Here's how the part is built. I have some questions about the finished solid (model axes, mm). A direction names the side the tool comes from. Round coordinates to 2 decimals unless told otherwise and drop trailing zeros. Write each loop counter-clockwise with the first axis right and the second up, starting at its lowest first coordinate (ties: lowest second). Pieces come first, ordered by that corner, then holes. Notation, with made-up numbers: M 79,-36.75 L 119,-36.75 A36 ccw 119,-2.75 Z; hole C -39,46.25 d9. An arc over 180 degrees is marked long. Use a Markdown table: item, result. Add a question column.
```python
from build123d import *

# Parameters (mm, degrees)
F1_DEPTH = 85.57783
F2_W     = 470.658332
F2_H     = 132.007137
F3_DEPTH = 332.33001
F4_R     = 3.175
F5_DEPTH = 369.06305


with BuildPart() as f1:
    # F0 (on Front) → F1 (new body)
    with BuildSketch(Plane.XZ):
        with BuildLine():
            ThreePointArc((-209.55, 0), (0, 209.55), (209.55, 0))
            Line((209.55, 0), (214.597345, 0))
            ThreePointArc((214.597345, 0), (0, 214.597345), (-214.597345, 0))
            Line((-214.597345, 0), (-209.55, 0))
        make_face()
    extrude(amount=F1_DEPTH)

    # F2 (on Top) → F3 (cut)
    with BuildSketch(Plane.XY):
        with Locations((5.359113, -37.707031)):
            Rectangle(F2_W, F2_H)
        Polygon((-61.859035, -72.326824), (-61.859035, -21.526824), (-31.379035, -21.526824), (-17.515417, -38.048841), (0, -38.048841), (13.863618, -21.526824), (44.343618, -21.526824), (44.343618, -72.326824), (13.863618, -72.326824), (0, -55.804808), (-17.515417, -55.804808), (-31.379035, -72.326824), align=None, mode=Mode.SUBTRACT)
    extrude(amount=F3_DEPTH, mode=Mode.SUBTRACT)

    # F4 (on Top) → F5 (cut)
    with BuildSketch(Plane.XY):
        with Locations((-51.647099, -30.972526)):
            Circle(F4_R)
        with Locations((-51.647099, -64.446411)):
            Circle(F4_R)
        with Locations((-33.92563, -47.118752)):
            Circle(F4_R)
        with Locations((9.262242, -47.118752)):
            Circle(F4_R)
        with Locations((33.022132, -30.972526)):
            Circle(F4_R)
        with Locations((32.234513, -64.446411)):
            Circle(F4_R)
    extrude(amount=F5_DEPTH, mode=Mode.SUBTRACT)


solid = f1.part
```
Item 1: Imagine slicing it at D-D on x = -23.5. List the corners of the cut face in (y, z) for me.
Item 2: Imagine slicing it at B-B on y = -62.5. List the corners of the cut face in (x, z) for me, plus the area to 3 significant figures.
Item 3: For pin 1 Ø7.5 at (x, y) = (-33.93, -47.12) entering from +Z; pin 2 Ø1.5 at (x, z) = (-24, 206) entering from -Y; pin 3 Ø6.5 at (x, z) = (-9, 212.5) entering from +Y; pin 4 Ø1.7 at (x, z) = (-8, 211.5) entering from -Y, each with a flat end and sliding along its axis, tell me the tip position at first contact or that it passes through.
Item 4: If we mould it in two halves opening along Y, with no side actions, what happens to faces 4 (the face through (35.17, -65.66, 209.54)), 5 (the face through (29, -21.527, 209)), 6 (the face through (7.03, -64.18, 211.81))? For each: +Y half, -Y half, draft (parallel to the pull), parting line (faces both ways), or undercut.
Item 5: I need wall thicknesses on probe 1 along X at (y, z) = (-31, 203.25); probe 2 along Z at (x, y) = (-51, -69); probe 3 along Z at (x, y) = (-39, -24.5). Which ranges of each line are inside material? Lowest first, please. Write a range as from..to.
Item 6: Imagine slicing it at A-A on y = -25.5. List the corners of the cut face in (x, z) for me, plus the area to 3 significant figures.
Item 7: Imagine slicing it at C-C on y = -37. List the corners of the cut face in (x, z) for me.
Item 8: On a 3-axis mill with a long thin cutter (end or side, diameter ignored), from which of +Z, -Z, +X, -X, +Y, -Y can I reach the whole of each face in a straight line? I mean faces 1 (the face through (-9, -55.805, 212)), 2 (the face through (44.344, -47, 207)), 3 (the face through (-9, -38.049, 212)). Say none if no direction works.
The answers:
| question | item | result |
|---|---|---|
| 1 | outline | M -62.94,208.23 L -30.92,208.23 L -30.92,213.31 L -62.94,213.31 Z |
| 2 | outline | M -61.86,200.21 A209.55 cw -54.16,202.43 L -54.16,207.65 A214.6 ccw -61.86,205.49 Z; M -49.14,203.71 A209.55 cw -23.13,208.27 L -23.13,213.35 A214.6 ccw -49.14,208.9 Z; M 5.62,209.47 A209.55 cw 29.73,207.43 L 29.73,212.53 A214.6 ccw 5.62,214.52 Z; M 34.74,206.65 A209.55 cw 44.34,204.8 L 44.34,209.97 A214.6 ccw 34.74,211.77 Z |
| 2 | area | 345 mm² |
| 3 | pin 1 | z = 212.46 |
| 3 | pin 2 | through |
| 3 | pin 3 | y = -38.05 |
| 3 | pin 4 | y = -55.8 |
| 4 | face 4 | undercut |
| 4 | face 5 | +Y half |
| 4 | face 6 | -Y half |
| 5 | probe 1 | -61.86..-54.82 |
| 5 | probe 2 | 203.25..208.45 |
| 5 | probe 3 | 205.89..211.02 |
| 6 | outline | M -61.86,200.21 A209.55 cw -28.05,207.66 L -28.05,212.76 A214.6 ccw -61.86,205.49 Z; M 10.53,209.29 A209.55 cw 44.34,204.8 L 44.34,209.97 A214.6 ccw 10.53,214.34 Z |
| 6 | area | 347 mm² |
| 7 | outline | M -61.86,200.21 A209.55 cw -18.4,208.74 L -18.4,213.81 A214.6 ccw -61.86,205.49 Z; M 0.88,209.55 A209.55 cw 44.34,204.8 L 44.34,209.97 A214.6 ccw 0.88,214.6 Z |
| 8 | face 1 | +Z, -Z, -Y |
| 8 | face 2 | +Z, -Z, +X, +Y, -Y |
| 8 | face 3 | +Z, -Z, +Y |
